```python
from build123d import *

# Parameters (mm, degrees)
RESSALTO_EXTRUS_O1_DEPTH = 1.75
ESBO_O2_R                = 3.3
CORTE_EXTRUS_O1_DEPTH    = 42.161268202
FILETE1_R                = 3


with BuildPart() as part:
    # Esboço1 → Ressalto-extrusão1 (new, symmetric)
    with BuildSketch(Plane.XY):
        Polygon((29, -9), (-9, 29), (-29, 29), (-29, -29), (29, -29), align=None)
    extrude(amount=RESSALTO_EXTRUS_O1_DEPTH, both=True)

    # Esboço2 → Corte-extrusão1 (cut, through all)
    with BuildSketch(Plane.XY.offset(1.75)):
        with Locations((-19, -19)):
            Circle(ESBO_O2_R)
        with Locations((1, -19)):
            Circle(ESBO_O2_R)
        with Locations((21, -19)):
            Circle(ESBO_O2_R)
        with Locations((-19, 1)):
            Circle(ESBO_O2_R)
        with Locations((-19, 21)):
            Circle(ESBO_O2_R)
    extrude(amount=-CORTE_EXTRUS_O1_DEPTH, mode=Mode.SUBTRACT)

    # Filete1
    filete1_edges = [part.edges().sort_by_distance(p)[0] for p in [
        (29, -29, 0),
        (-29, -29, 0),
        (-29, 29, 0),
        (-9, 29, 0),
        (29, -9, 0),
    ]]
    fillet(filete1_edges, radius=FILETE1_R)


solid = part.part
```
Geometry check sheet. Reference: the model listing, model coordinates, mm. Round coordinates to 2 decimals unless told otherwise and drop trailing zeros. Loops run counter-clockwise (first coordinate to the right, second up) from the corner with the lowest first, then second, coordinate; pieces in that order, holes last. Notation, with made-up numbers: (65.25, 21) - (98.25, 21) arc R21 ccw to (98.25, 49) - close; hole circle Ø7 at (50, 57.5). An arc over 180 degrees is marked (long way). Write each question's results on one line, items separated by ' | '. Start each with the question number.
Q1. Thickness scan on line 1 (Y direction, x = -19, z = 0.7); line 2 (Y direction, x = 24, z = -1.05); line 3 (X direction, y = -21, z = -1.6). Record the ranges inside material, lowest first. Write a range as [from, to].
Q2. Cross-section at B-B on x = 21. Enter the section's corners in (y, z), and give its area (3 significant figures).
Q3. Gauge pin test, flat ends, axial feed: P1, Ø10.5, axis at x = 1, y = -19, coming from the -Z side; P2, Ø1, axis at x = -2, z = 0.5, coming from the +Y side; P3, Ø1, axis at y = -5, z = 0.5, coming from the +X side. Record the tip position at first contact, or that the pin passes through.
Q4. Cross-section at D-D on y = 1. Enter the section's corners in (x, z), and give its area (3 significant figures).
Q5. Release check for a two-part mould opening along Y. For faces 1 (the flat face through (-7, -6, 1.75)), 2 (the cylindrical face through (28.14, -28.1, -0.02)), 3 (the cylindrical face through (-22.3, 1.1, 0)) record: +Y half, -Y half, draft (parallel to the pull), parting line (faces both ways), or undercut.
Q6. Cross-section at C-C on z = 1.2. Enter the section's corners in (x, y).
Q7. Cross-section at A-A on y = -19. Enter the section's corners in (x, z), and give its area (3 significant figures).
Answers below:
1) line 1: y = [-29, -22.3], [-15.7, -2.3], [4.3, 17.7], [24.3, 29] | line 2: y = [-29, -20.37], [-17.63, -4] | line 3: x = [-29, -21.62], [-16.38, -1.62], [3.62, 18.38], [23.62, 29]
2) outline: (-29, -1.75) - (-22.3, -1.75) - (-22.3, 1.75) - (-29, 1.75) - close; (-15.7, -1.75) - (-1, -1.75) - (-1, 1.75) - (-15.7, 1.75) - close | area: 74.9 mm²
3) P1: stops at z = -1.75 | P2: stops at y = 22.5 | P3: stops at x = 25.5
4) outline: (-29, -1.75) - (-22.3, -1.75) - (-22.3, 1.75) - (-29, 1.75) - close; (-15.7, -1.75) - (19, -1.75) - (19, 1.75) - (-15.7, 1.75) - close | area: 145 mm²
5) face 1: draft | face 2: -Y half | face 3: undercut
6) outline: (-29, -26) arc R3 ccw to (-26, -29) - (26, -29) arc R3 ccw to (29, -26) - (29, -10.24) arc R3 ccw to (28.12, -8.12) - (-8.12, 28.12) arc R3 ccw to (-10.24, 29) - (-26, 29) arc R3 ccw to (-29, 26) - close; hole circle Ø6.6 at (-19, -19); hole circle Ø6.6 at (-19, 1); hole circle Ø6.6 at (-19, 21); hole circle Ø6.6 at (1, -19); hole circle Ø6.6 at (21, -19)
7) outline: (-29, -1.75) - (-22.3, -1.75) - (-22.3, 1.75) - (-29, 1.75) - close; (-15.7, -1.75) - (-2.3, -1.75) - (-2.3, 1.75) - (-15.7, 1.75) - close; (4.3, -1.75) - (17.7, -1.75) - (17.7, 1.75) - (4.3, 1.75) - close; (24.3, -1.75) - (29, -1.75) - (29, 1.75) - (24.3, 1.75) - close | area: 134 mm²
